Geometry check sheet. Reference: the model listing, model coordinates, mm. A direction names the side the tool comes from. Coordinates: 2 decimals unless noted, no trailing zeros. Write each loop counter-clockwise with the first axis right and the second up, starting at its lowest first coordinate (ties: lowest second). Pieces come first, ordered by that corner, then holes. Notation, with made-up numbers: (-25, 35.25) -> (32, 35.25) arc R36 ccw to (32, 69.25) -> close; hole circle Ø5 at (83.25, -14.75). An arc over 180 degrees is marked (long way). One line per question, with ' | ' between items.
from build123d import *

# Parameters (mm, degrees)
BOSS_EXTRUDE2_DEPTH = 68.5
SKETCH4_R           = 4
CUT_EXTRUDE1_DEPTH  = 6
SKETCH5_R           = 2.5
CUT_EXTRUDE2_DEPTH  = 4
SKETCH7_W           = 20
SKETCH7_H           = 2.5
BOSS_EXTRUDE6_DEPTH = 3
FILLET2_R           = 5


with BuildPart() as part:
    # Sketch1 → Boss-Extrude2 (new body, symmetric)
    with BuildSketch(Plane.XY):
        Polygon((-7, 4.5), (7, 4.5), (7, 2), (4.5, 2), (4.5, -2), (10, -2), (10, -4.5), (-10, -4.5), (-10, -2), (-4.5, -2), (-4.5, 2), (-7, 2), align=None)
    extrude(amount=BOSS_EXTRUDE2_DEPTH, both=True)

    # Sketch4 → Cut-Extrude1 (cut)
    with BuildSketch(Plane(origin=(0, 4.5, 0), x_dir=(1, 0, 0), z_dir=(0, 1, 0))):
        Circle(SKETCH4_R)
        with Locations((0, 40)):
            Circle(SKETCH4_R)
        with Locations((0, -40)):
            Circle(SKETCH4_R)
    extrude(amount=-CUT_EXTRUDE1_DEPTH, mode=Mode.SUBTRACT)

    # Sketch5 → Cut-Extrude2 (cut)
    with BuildSketch(Plane(origin=(0, -1.5, 0), x_dir=(1, 0, 0), z_dir=(0, 1, 0))):
        with Locations((0, 40)):
            Circle(SKETCH5_R)
        Circle(SKETCH5_R)
        with Locations((0, -40)):
            Circle(SKETCH5_R)
    extrude(amount=-CUT_EXTRUDE2_DEPTH, mode=Mode.SUBTRACT)

    # Sketch7 → Boss-Extrude6 (add)
    with BuildSketch(Plane.XY.offset(68.5)):
        with Locations((0, -3.25)):
            Rectangle(SKETCH7_W, SKETCH7_H)
    extrude(amount=BOSS_EXTRUDE6_DEPTH)

    # Fillet2
    fillet2_edges = [part.edges().sort_by_distance(p)[0] for p in [
        (10, -3.25, -68.5),
        (10, -3.25, 71.5),
    ]]
    fillet(fillet2_edges, radius=FILLET2_R)


solid = part.part
1. Mould release check, pull along Z, two halves, no side actions. Record for faces 4 (the face through (-4.5, 0, 1)), 5 (the face through (-0.521, 1.542, 36.034)), 6 (the face through (8.57, -3.23, 70)): released by +Z, released by -Z, zero draft, split by the parting line, or undercut.
Worked answers:
face 4: zero draft | face 5: undercut | face 6: released by +Z
2. Go/stop test with flat-tipped pins: P1, Ø4.5, axis at x = 0, z = 0, coming from the -Y side; P2, Ø0.8, axis at y = 3.5, z = 10.5, coming from the +X side; P3, Ø2, axis at y = 0.5, z = -11.5, coming from the +X side; P4, Ø2, axis at y = 2.5, z = 19.5, coming from the -X side. Record where each tip stops, or that it passes through.
Worked answers:
P1: through | P2: x = 7 | P3: x = 4.5 | P4: x = -7
3. Cross-section at A-A on z = 0. Record the boundary of the cut face in (x, y), and give its area (3 significant figures).
Worked answers:
outline: (-10, -4.5) -> (-2.5, -4.5) -> (-2.5, -1.5) -> (-4, -1.5) -> (-4, 4.5) -> (-7, 4.5) -> (-7, 2) -> (-4.5, 2) -> (-4.5, -2) -> (-10, -2) -> close; (2.5, -4.5) -> (10, -4.5) -> (10, -2) -> (4.5, -2) -> (4.5, 2) -> (7, 2) -> (7, 4.5) -> (4, 4.5) -> (4, -1.5) -> (2.5, -1.5) -> close | area: 58.0 mm²
4. Material ranges on line 1 (Z direction, x = 0, y = -2.35); line 2 (X direction, y = -3.9, z = 40); line 3 (Y direction, x = 6, z = -0.5), recorded low to high. Write a range as from..to.
Worked answers:
line 1: -68.5..-42.5, -37.5..-2.5, 2.5..37.5, 42.5..71.5 | line 2: -10..-2.5, 2.5..10 | line 3: -4.5..-2, 2..4.5
5. Cross-section at B-B on x = 0. Give the number of separate pieces and of enclosed holes in the cut face, and give its area (3 significant figures).
Worked answers:
separate pieces: 4 | enclosed holes: 0 | area: 1,050 mm²
6. Cross-section at C-C on z = 24. Record the boundary of the cut face in (x, y), and give its area (3 significant figures).
Worked answers:
outline: (-10, -4.5) -> (10, -4.5) -> (10, -2) -> (4.5, -2) -> (4.5, 2) -> (7, 2) -> (7, 4.5) -> (-7, 4.5) -> (-7, 2) -> (-4.5, 2) -> (-4.5, -2) -> (-10, -2) -> close | area: 121 mm²
7. Tool access check on faces 1 (the face through (6, 2, 1)), 2 (the face through (8.57, -3.27, -67)), 3 (the face through (2, -1.5, 38)). Record the directions out of +Z, -Z, +X, -X, +Y, -Y that give a thin tool (end or side, any length) a straight path to the whole face; none if there is none.
Worked answers:
face 1: +Z, -Z, +X | face 2: -Z, +X, -Y | face 3: +Y
